Part print with two shaded views. Sizes in mm from the minimum x, y, z corner. A direction names the side the tool comes from. Coordinates: 2 decimals unless noted, no trailing zeros. Loops run counter-clockwise (first coordinate to the right, second up) from the corner with the lowest first, then second, coordinate; pieces in that order, holes last. Notation, with made-up numbers: M 13.5,-4 L 61.5,-4 A38 ccw 61.5,35 Z; hole C 32,3 d6. An arc over 180 degrees is marked long. Write item = value, one per line. Start each with the question number.
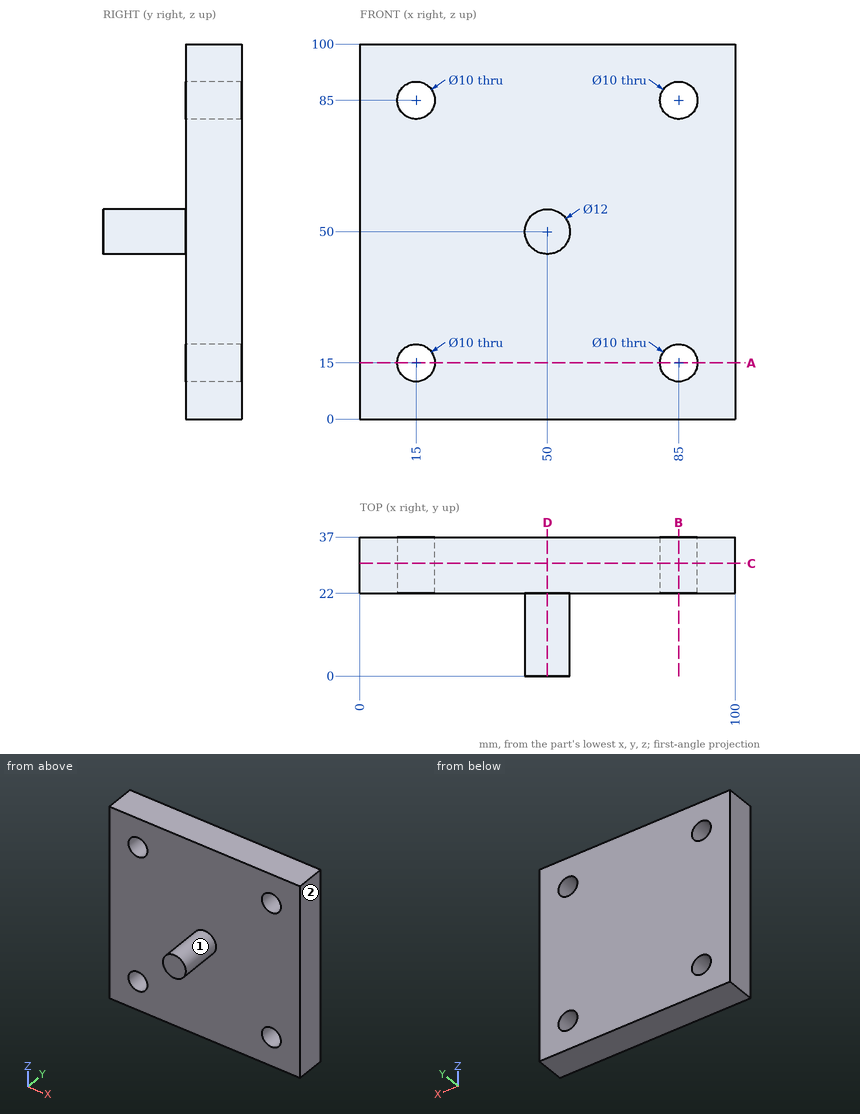
Item 1: Cut at A-A (z = 15). Give the cut face in (x, y), plus the area to 3 significant figures.
Item 2: Cut at B-B (x = 85). Give the cut face in (y, z), plus the area to 3 significant figures.
Item 3: Probe L1, parallel to Z at x = 15, y = 28.25; L2, parallel to Y at x = 34, z = 89. List the from-to ranges inside material, lowest first.
Item 4: 3-axis set-ups, long thin cutter, end or side, ignore diameter. For the marked faces 1 and 2: which of +Z, -Z, +X, -X, +Y, -Y reach the whole face in a straight line?
Item 5: Cut at D-D (x = 50). Give the cut face in (y, z).
Item 6: Pin check, flat tips, straight feed: pin 1 Ø13 at (x, z) = (15, 85) entering from -Y; pin 2 Ø9 at (x, z) = (85, 15) entering from -Y. Stop position of each tip, or through.
Item 7: Cut at C-C (y = 30). Give the cut face in (x, z), plus the area to 3 significant figures.
Reported:
q1.outline = M 0,22 L 10,22 L 10,37 L 0,37 Z; M 20,22 L 80,22 L 80,37 L 20,37 Z; M 90,22 L 100,22 L 100,37 L 90,37 Z
q1.area = 1,200 mm^2
q2.outline = M 22,0 L 37,0 L 37,10 L 22,10 Z; M 22,20 L 37,20 L 37,80 L 22,80 Z; M 22,90 L 37,90 L 37,100 L 22,100 Z
q2.area = 1,200 mm^2
q3.L1 = 0 to 10, 20 to 80, 90 to 100
q3.L2 = 22 to 37
q4.face_1 = -Y
q4.face_2 = +Z, -Z, +X, +Y, -Y
q5.outline = M 0,44 L 22,44 L 22,0 L 37,0 L 37,100 L 22,100 L 22,56 L 0,56 Z
q6.pin_1 = 22
q6.pin_2 = through
q7.outline = M 0,0 L 100,0 L 100,100 L 0,100 Z; hole C 15,15 d10; hole C 15,85 d10; hole C 85,15 d10; hole C 85,85 d10
q7.area = 9,690 mm^2
